```python
from build123d import *

# Parameters (mm, degrees)
ESQUISSE1_R                                     = 6
BOSS_EXTRU_1_DEPTH                              = 7
ESQUISSE2_OUTSIDE_W                             = 17.672
ESQUISSE2_OUTSIDE_H                             = 17.672
ESQUISSE2_OUTSIDE_R                             = 4.5
ENL_V_MAT_EXTRU_1_DEPTH                         = 1.5
CHANFREIN1_SIZE                                 = 1
CHAMBRAGE_POUR_VIS_T_TE_CYLINDRIQUE_D           = 3.2
CHAMBRAGE_POUR_VIS_T_TE_CYLINDRIQUE_CBORE_D     = 6.5
CHAMBRAGE_POUR_VIS_T_TE_CYLINDRIQUE_CBORE_DEPTH = 4
ENL_V_MAT_EXTRU_2_DEPTH                         = 12
R_P_TITION_CIRCULAIRE1_COUNT                    = 16


with BuildPart() as part:
    # Esquisse1 → Boss.-Extru.1 (new body)
    with BuildSketch(Plane(origin=(0, 0, 0), x_dir=(1, 0, 0), z_dir=(0, 1, 0))):
        with Locations(Location((0, 0, 0), (0, 0, 270))):
            Circle(ESQUISSE1_R)
    extrude(amount=BOSS_EXTRU_1_DEPTH)

    # Esquisse2 outside → Enlèv. mat.-Extru.1 (cut)
    with BuildSketch(Plane.XZ):
        Rectangle(ESQUISSE2_OUTSIDE_W, ESQUISSE2_OUTSIDE_H)
        with Locations(Location((0, 0, 0), (0, 0, 270))):
            Circle(ESQUISSE2_OUTSIDE_R, mode=Mode.SUBTRACT)
    extrude(amount=-ENL_V_MAT_EXTRU_1_DEPTH, mode=Mode.SUBTRACT)

    # Chanfrein1
    chanfrein1_edges = [part.edges().sort_by_distance(p)[0] for p in [
        (0, 7, -6),
        (0, 1.5, -6),
    ]]
    chamfer(chanfrein1_edges, length=CHANFREIN1_SIZE)

    # Chambrage pour vis à tête cylindrique à 6 pans creux (ou vis CHC) M31 (through all)
    with Locations(Plane(origin=(0, 7, 0), x_dir=(1, 0, 0), z_dir=(0, 1, 0))):
        with Locations((0, 0)):
            CounterBoreHole(CHAMBRAGE_POUR_VIS_T_TE_CYLINDRIQUE_D / 2, CHAMBRAGE_POUR_VIS_T_TE_CYLINDRIQUE_CBORE_D / 2, CHAMBRAGE_POUR_VIS_T_TE_CYLINDRIQUE_CBORE_DEPTH)

    # Esquisse5 → Enlèv. mat.-Extru.2 (cut, through all)
    with BuildSketch(Plane(origin=(0, 7, 0), x_dir=(1, 0, 0), z_dir=(0, 1, 0))):
        Polygon((-5, 0), (-6.645642825, 1.380858287), (-6.645642825, -1.380858287), align=None)
    enl_v_mat_extru_2 = extrude(amount=-ENL_V_MAT_EXTRU_2_DEPTH, mode=Mode.SUBTRACT)

    # Répétition circulaire1: Enlèv. mat.-Extru.2 ×16 about axis
    r_p_tition_circulaire1_axis = Axis((0, 0, 0), (0, 1, 0))
    for i in range(1, R_P_TITION_CIRCULAIRE1_COUNT):
        add(enl_v_mat_extru_2.rotate(r_p_tition_circulaire1_axis, i * 360 / R_P_TITION_CIRCULAIRE1_COUNT), mode=Mode.SUBTRACT)


solid = part.part
```
Could you check a few things on this model? Use its own coordinates, in mm. Give positions to 0.01 mm unless a question says otherwise; leave off trailing zeros. Use one line per item in the form item = value.
1. I'm going to push flat-ended pins straight in: pin 1 Ø7 at (x, z) = (1.5, 0.5) entering from +Y; pin 2 Ø2 at (x, y) = (-3.5, 4) entering from -Z; pin 3 Ø1 at (y, z) = (6, 4) entering from +X; pin 4 Ø5 at (x, z) = (0, 0) entering from +Y. Where does each tip first touch, or does it pass through?
Response values:
pin_1 = 7
pin_2 = -5.19
pin_3 = 4.87
pin_4 = 3
2. Thinking about a two-plate mould opening in Z: for faces 1 (the face through (-4.48, 1.88, -2.98)), 2 (the face through (1.27, 1.48, 0.97)), 3 (the face through (1.352, 0.74, -4.292)), 4 (the face through (3.59, 4.29, 4.14)), which applies, released by +Z, released by -Z, zero draft, split by the parting line, or undercut?
Response values:
face_1 = released by -Z
face_2 = undercut
face_3 = split by the parting line
face_4 = undercut
3. I need wall thicknesses on probe 1 along Y at (x, z) = (4.5, 2); probe 2 along Y at (x, z) = (1, -1.75); probe 3 along Z at (x, y) = (1, 4). Which ranges of each line are inside material? Lowest first, please.
Response values:
probe_1 = 1.5 to 7
probe_2 = 0 to 3
probe_3 = -5.92 to -3.09, 3.09 to 5.92
